Build history of the part. All positions in model axes, mm. A direction names the side the tool comes from. Round coordinates to 2 decimals unless told otherwise and drop trailing zeros. Write each loop counter-clockwise with the first axis right and the second up, starting at its lowest first coordinate (ties: lowest second). Pieces come first, ordered by that corner, then holes.
1) Pull direction Y, two halves, no side cores. Call faces 4 (the flat face through (1, 3.49, 20)), 5 (the flat face through (1, -5, 30.127)), 6 (the flat face through (1, 6.49, 23)): +Y half, -Y half, draft (parallel to the pull), parting line (faces both ways), or undercut.
2) Saw through at B-B (y = 4.5). Write the cut outline in (x, z), plus the area to 3 significant figures.
3) Which spindle directions (+Z, -Z, +X, -X, +Y, -Y) get a long thin tool onto all of the face, cutting with end or side? Do faces 1 (the flat face through (1, -3.51, 27)), 2 (the cylindrical face through (1.479, 43.636, 5.826)), 3 (the flat face through (1, 3.49, 25)). Say none if no direction does.
4) Wall check: probe 1 along Z at (x, y) = (0.5, 24.5); probe 2 along Z at (x, y) = (1.25, 0); probe 3 along Y at (x, z) = (0.35, 24.5). Give the ranges that are in metal, low to high.
5) Saw through at C-C (z = 10.5). Write the cut outline in (x, y), plus the area to 3 significant figures.
6) Saw through at D-D (x = 2.05). State how many separate pieces and enclosed holes the cut face has, plus the area to 3 significant figures.
7) Flat gauge pins, fed straight in: pin 1 (10 mm diameter, centred on y = 38, z = 11.5, fed in from -X); pin 2 (0.9 mm diameter, centred on x = 1.5, y = 2, fed in from +Z); pin 3 (0.9 mm diameter, centred on x = 1.5, y = 4.5, fed in from +Z); pin 4 (0.6 mm diameter, centred on x = 1.5, z = 20.5, fed in from +Y). Where does each tip first touch, or does it go through?
8) Saw through at A-A (y = 37). Write the cut outline in (x, z), plus the area to 3 significant figures.
from build123d import *

# Parameters (mm, degrees)
F0_R     = 1.6
F1_DEPTH = 3


# Not quite as in the source:
# - ends of sketch curves that miss each other by under 0.0002 mm in the source are joined


with BuildPart() as f1:
    # F0 (on Right) → F1 (new body)
    with BuildSketch(Plane.YZ):
        with BuildLine():
            Line((6.490295, 24.126887), (6.490295, 20.926875))
            Line((6.490295, 20.926875), (3.490295, 20.926875))
            Line((3.490295, 20.926875), (3.490295, 19.651881))
            Line((3.490295, 19.651881), (-0.509733, 19.651881))
            Line((-0.509733, 19.651881), (-0.509733, 20.926875))
            Line((-0.509733, 20.926875), (-3.509705, 20.926875))
            Line((-3.509705, 20.926875), (-3.509702, 15.792903))
            ThreePointArc((-3.509702, 15.792903), (-3.4427150061, 15.542903527), (-3.2597030539, 15.3598909066))
            ThreePointArc((-3.2597030539, 15.3598909066), (-3.1561520924, 14.5733251264), (-3.9427177764, 14.6768791291))
            ThreePointArc((-3.9427177764, 14.6768791291), (-4.1257299355, 14.8598916646), (-4.37573, 14.926879))
            Line((-4.37573, 14.926879), (-6.009757, 14.926882))
            ThreePointArc((-6.009757, 14.926882), (-6.3633103906, 14.7804353906), (-6.509757, 14.426882))
            Line((-6.509757, 14.426882), (-6.509757, 9.426885))
            ThreePointArc((-6.509757, 9.426885), (-6.3633103906, 9.0733316094), (-6.009757, 8.926885))
            Line((-6.009757, 8.926885), (-4.375728, 8.926885))
            ThreePointArc((-4.375728, 8.926885), (-4.125728527, 8.9938719939), (-3.9427159066, 9.1768839461))
            ThreePointArc((-3.9427159066, 9.1768839461), (-3.1561511264, 9.2804349076), (-3.2597051291, 8.4938692236))
            ThreePointArc((-3.2597051291, 8.4938692236), (-3.4427176646, 8.3108560645), (-3.509705, 8.060856))
            Line((-3.509705, 8.060856), (-3.509702, 3.526887))
            Line((-3.509702, 3.526887), (0, 0))
            ThreePointArc((0, 0), (1.6251015018, -1.0901687381), (3.544158, -1.473111))
            Line((3.544158, -1.473111), (42.206461, -1.47311))
            ThreePointArc((42.206461, -1.47311), (43.6206745624, -0.8873235624), (44.206461, 0.52689))
            Line((44.206461, 0.52689), (44.206463, 4.426926))
            ThreePointArc((44.206463, 4.426926), (43.6206765624, 5.8411395624), (42.206463, 6.426926))
            Line((42.206463, 6.426926), (24.990243, 6.426926))
            ThreePointArc((24.990243, 6.426926), (13.890243, 17.526926), (24.990243, 28.626926))
            Line((24.990243, 28.626926), (42.206463, 28.626926))
            ThreePointArc((42.206463, 28.626926), (43.6206765624, 29.2127124376), (44.206463, 30.626926))
            Line((44.206463, 30.626926), (44.206463, 34.526876))
            ThreePointArc((44.206463, 34.526876), (43.6206745624, 35.9410875624), (42.206461, 36.526874))
            Line((42.206461, 36.526874), (8.985147, 36.526873))
            ThreePointArc((8.985147, 36.526873), (7.141367531, 36.8792416388), (5.5574640867, 37.8866820921))
            Line((5.5574640867, 37.8866820921), (3.135704, 40.167064))
            ThreePointArc((3.135704, 40.167064), (1.551800469, 41.1745043612), (-0.291979, 41.526873))
            Line((-0.291979, 41.526873), (-3.509705, 41.526873))
            Line((-3.509705, 41.526873), (-3.509702, 36.992904))
            ThreePointArc((-3.509702, 36.992904), (-3.4427150061, 36.742904527), (-3.2597030539, 36.5598919066))
            ThreePointArc((-3.2597030539, 36.5598919066), (-3.1561520924, 35.7733261264), (-3.9427177764, 35.8768801291))
            ThreePointArc((-3.9427177764, 35.8768801291), (-4.1257299355, 36.0598926646), (-4.37573, 36.12688))
            Line((-4.37573, 36.12688), (-6.009757, 36.126883))
            ThreePointArc((-6.009757, 36.126883), (-6.3633103906, 35.9804363906), (-6.509757, 35.626883))
            Line((-6.509757, 35.626883), (-6.509757, 30.626886))
            ThreePointArc((-6.509757, 30.626886), (-6.3633103906, 30.2733326094), (-6.009757, 30.126886))
            Line((-6.009757, 30.126886), (-4.375728, 30.126886))
            ThreePointArc((-4.375728, 30.126886), (-4.125728527, 30.1938729939), (-3.9427159066, 30.3768849461))
            ThreePointArc((-3.9427159066, 30.3768849461), (-3.1561511264, 30.4804359076), (-3.2597051291, 29.6938702236))
            ThreePointArc((-3.2597051291, 29.6938702236), (-3.4427176646, 29.5108580645), (-3.509705, 29.260858))
            Line((-3.509705, 29.260858), (-3.509705, 24.126887))
            Line((-3.509705, 24.126887), (-0.509733, 24.126887))
            Line((-0.509733, 24.126887), (-0.509733, 25.401881))
            Line((-0.509733, 25.401881), (3.490295, 25.401881))
            Line((3.490295, 25.401881), (3.490295, 24.126887))
            Line((3.490295, 24.126887), (6.490295, 24.126887))
        make_face()
        with Locations((9.490194, 2.026885)):
            Circle(F0_R, mode=Mode.SUBTRACT)
        with Locations((40.490194, 2.026885)):
            Circle(F0_R, mode=Mode.SUBTRACT)
        with Locations((9.490194, 33.026885)):
            Circle(F0_R, mode=Mode.SUBTRACT)
        with Locations((40.490194, 33.026885)):
            Circle(F0_R, mode=Mode.SUBTRACT)
    extrude(amount=F1_DEPTH)


solid = f1.part
Evaluation:
1. face 4: undercut
1. face 5: draft
1. face 6: -Y half
2. outline: (0, -1.47) - (3, -1.47) - (3, 20.93) - (0, 20.93) - close; (0, 24.13) - (3, 24.13) - (3, 38.88) - (0, 38.88) - close
2. area: 111 mm2
3. face 1: +X, -X, -Y
3. face 2: +X, -X, +Y
3. face 3: +X, -X
4. probe 1: z = -1.47 to 6.44, 28.62 to 36.53
4. probe 2: z = 0 to 19.65, 25.4 to 41.52
4. probe 3: y = -3.51 to -0.51, 3.49 to 16.35
5. outline: (0, -6.51) - (3, -6.51) - (3, 16.4) - (0, 16.4) - close
5. area: 68.7 mm2
6. separate pieces: 1
6. enclosed holes: 4
6. area: 1,170 mm2
7. pin 1: passes through
7. pin 2: stops at z = 41.18
7. pin 3: stops at z = 39.31
7. pin 4: stops at y = 14.38
8. outline: (0, -1.47) - (3, -1.47) - (3, 6.43) - (0, 6.43) - close; (0, 28.63) - (3, 28.63) - (3, 36.53) - (0, 36.53) - close
8. area: 47.4 mm2
